Source: CAD feature listing. Evaluate the final solid. Frame: model axes, mm. A direction names the side the tool comes from. Give positions to 0.01 mm unless a question says otherwise; leave off trailing zeros. Order: outer loops, then holes, each group sorted by start corner. A loop starts at its lowest first (then second) coordinate and runs counter-clockwise, first axis right, second up.
```python
from build123d import *

# Parameters (mm, degrees)
F0_W     = 114.3
F0_H     = 152.4
F1_DEPTH = 101.6
F2_W     = 50.8
F2_H     = 50.8
F3_DEPTH = 38.1
F5_DEPTH = 63.5


with BuildPart() as f1:
    # F0 (on Top) → F1 (new body)
    with BuildSketch(Plane.XY):
        with Locations((-6.724683, 26.519689)):
            Rectangle(F0_W, F0_H)
    extrude(amount=F1_DEPTH)

    # F2 (on face) → F3 (cut)
    with BuildSketch(Plane.XY.offset(101.6)):
        with Locations((-6.183666, 66.633569)):
            Rectangle(F2_W, F2_H)
    extrude(amount=-F3_DEPTH, mode=Mode.SUBTRACT)

    # F4 (on face) → F5 (cut)
    with BuildSketch(Plane.XY.offset(101.6)):
        Polygon((19.216334, 41.233569), (-31.583666, 41.233569), (-36.934618, 41.233569), (-36.934618, -23.049315), (26.324298, -23.049315), (26.324298, 41.233569), align=None)
    extrude(amount=-F5_DEPTH, mode=Mode.SUBTRACT)


solid = f1.part
```
1) Section query B-B, the plane y = 38. Return the cut outline in (x, z).
Report:
outline: (-63.87, 0) - (50.43, 0) - (50.43, 101.6) - (26.32, 101.6) - (26.32, 38.1) - (-36.93, 38.1) - (-36.93, 101.6) - (-63.87, 101.6) - close
2) Draft query along Y for faces 1 (the flat face through (-8, 28, 0)), 2 (the flat face through (-7, 92.034, 83)), 3 (the flat face through (-8, -49.68, 50)), 4 (the flat face through (-7, 67, 63.5)). Return one class per face: +Y half, -Y half, draft (parallel to the pull), parting line (faces both ways), or undercut.
Report:
face 1: draft
face 2: undercut
face 3: -Y half
face 4: undercut
3) Section query D-D, the plane z = 84. Return the cut outline in (x, y), and give its area (3 significant figures).
Report:
outline: (-63.87, -49.68) - (50.43, -49.68) - (50.43, 102.72) - (-63.87, 102.72) - close; hole (-36.93, -23.05) - (26.32, -23.05) - (26.32, 41.23) - (19.22, 41.23) - (19.22, 92.03) - (-31.58, 92.03) - (-31.58, 41.23) - (-36.93, 41.23) - close
area: 10,800 mm2
4) Section query C-C, the plane x = -9. Return the cut outline in (y, z), and give its area (3 significant figures).
Report:
outline: (-49.68, 0) - (102.72, 0) - (102.72, 101.6) - (92.03, 101.6) - (92.03, 63.5) - (41.23, 63.5) - (41.23, 38.1) - (-23.05, 38.1) - (-23.05, 101.6) - (-49.68, 101.6) - close
area: 9,470 mm2
5) Material intervals for L1, parallel to Y at x = -14, z = 97.5; L2, parallel to X at y = -1.5, z = 96.5; L3, parallel to X at y = 72, z = 71, sorted ascending.
Report:
L1: y = -49.68 to -23.05, 92.03 to 102.72
L2: x = -63.87 to -36.93, 26.32 to 50.43
L3: x = -63.87 to -31.58, 19.22 to 50.43
6) Section query A-A, the plane z = 53.5. Return the cut outline in (x, y).
Report:
outline: (-63.87, -49.68) - (50.43, -49.68) - (50.43, 102.72) - (-63.87, 102.72) - close; hole (-36.93, -23.05) - (26.32, -23.05) - (26.32, 41.23) - (-36.93, 41.23) - close
7) Pin query (flat end, axial travel): pin 1 (1.5 mm diameter, centred on x = 24, y = -19.5, fed in from +Z); pin 2 (3 mm diameter, centred on x = 38, y = 42.5, fed in from -Z). Return the tip coordinate at first contact, or that it passes through.
Report:
pin 1: stops at z = 38.1
pin 2: stops at z = 0
8) Reachability of faces 5 (the flat face through (-36.935, 10, 70)), 6 (the flat face through (-33, 45, 101.6)) from +Z, -Z, +X, -X, +Y, -Y: full face, straight path, thin tool, end or side. Return the list, or none.
Report:
face 5: +Z
face 6: +Z, +X, -X, +Y, -Y
